```python
from build123d import *

# Parameters (mm, degrees)
BOSS_EXTRUDE1_DEPTH = 2
SKETCH3_R           = 35.7
BOSS_EXTRUDE2_DEPTH = 18.5
SKETCH5_W           = 12
SKETCH5_H           = 10
SKETCH5_R           = 1.75
BOSS_EXTRUDE3_DEPTH = 18.5
SKETCH6_R           = 36.4
BOSS_EXTRUDE5_DEPTH = 18.5
BOSS_EXTRUDE6_DEPTH = 21.5
SKETCH8_W           = 12.454054054
SKETCH8_H           = 5
CUT_EXTRUDE1_DEPTH  = 12
SKETCH9_W           = 10
SKETCH9_H           = 3
CUT_EXTRUDE2_DEPTH  = 21
CHAMFER1_SIZE       = 0.5
FILLET1_R           = 2
CHAMFER2_SIZE       = 2
SKETCH10_W          = 14
SKETCH10_H          = 10
CUT_EXTRUDE3_DEPTH  = 13


# Some blends are built 0.0001 mm under size
with BuildPart() as part:
    # Sketch4 → Boss-Extrude1 (new body)
    with BuildSketch(Plane(origin=(0, 0, 0), x_dir=(1, 0, 0), z_dir=(0, 1, 0))):
        with BuildLine():
            Line((37, 0), (37, -58))
            Line((37, -58), (-37, -58))
            Line((-37, -58), (-37, 0))
            ThreePointArc((-37, 0), (0, 37), (37, 0))
        make_face()
        with BuildLine():
            Line((-11.5, 6.062177826), (-24.769230769, 13.056998396))
            ThreePointArc((-24.769230769, 13.056998396), (-20.089945679, 19.503694076), (-13.784615385, 24.371794737))
            Line((-13.784615385, 24.371794737), (-6.4, 11.315476128))
            ThreePointArc((-6.4, 11.315476128), (-9.327474779, 9.055286535), (-11.5, 6.062177826))
        make_face(mode=Mode.SUBTRACT)
    extrude(amount=BOSS_EXTRUDE1_DEPTH)

    # Sketch3 → Boss-Extrude2 (add)
    with BuildSketch(Plane(origin=(0, 0, 0), x_dir=(1, 0, 0), z_dir=(0, 1, 0))):
        with BuildLine():
            Line((-37, 0), (-37, -58))
            Line((-37, -58), (-35, -58))
            Line((-35, -58), (-35, -38))
            Line((-35, -38), (35, -38))
            Line((35, -38), (35, -58))
            Line((35, -58), (37, -58))
            Line((37, -58), (37, 0))
            ThreePointArc((37, 0), (0, 37), (-37, 0))
        make_face()
        with Locations(Location((0, 0, 0), (0, 0, 270))):
            Circle(SKETCH3_R, mode=Mode.SUBTRACT)
    extrude(amount=BOSS_EXTRUDE2_DEPTH)

    # Sketch5 → Boss-Extrude3 (add)
    with BuildSketch(Plane(origin=(0, 0, 0), x_dir=(1, 0, 0), z_dir=(0, 1, 0))):
        with Locations((0, 40.7)):
            Rectangle(SKETCH5_W, SKETCH5_H)
        with Locations(Location((0, 41.35, 0), (0, 0, 270))):
            Circle(SKETCH5_R, mode=Mode.SUBTRACT)
    extrude(amount=BOSS_EXTRUDE3_DEPTH)

    # Sketch6 → Boss-Extrude5 (add)
    with BuildSketch(Plane(origin=(0, 0, 0), x_dir=(-1, 0, 0), z_dir=(0, 1, 0))):
        with BuildLine():
            Line((37.4, 0), (37.4, 58))
            Line((37.4, 58), (35, 58))
            Line((35, 58), (35, 38))
            Line((35, 38), (-35, 38))
            Line((-35, 38), (-35, 58))
            Line((-35, 58), (-37.4, 58))
            Line((-37.4, 58), (-37.4, 0))
            ThreePointArc((-37.4, 0), (-28.50952425, -24.206755814), (-6.064864865, -36.904978176))
            Line((-6.064864865, -36.904978176), (6.064864865, -36.904978176))
            ThreePointArc((6.064864865, -36.904978176), (28.50952425, -24.206755814), (37.4, 0))
        make_face()
        Circle(SKETCH6_R, mode=Mode.SUBTRACT)
    extrude(amount=BOSS_EXTRUDE5_DEPTH)

    # Sketch7 → Boss-Extrude6 (add)
    with BuildSketch(Plane(origin=(0, 0, 0), x_dir=(1, 0, 0), z_dir=(0, 1, 0))):
        with BuildLine():
            Line((37.4, 0), (37.4, -58))
            Line((37.4, -58), (38.4, -58))
            Line((38.4, -58), (38.4, 0))
            ThreePointArc((38.4, 0), (29.271810995, 24.853995274), (6.227027027, 37.891742298))
            Line((6.227027027, 37.891742298), (-6.227027027, 37.891742298))
            ThreePointArc((-6.227027027, 37.891742298), (-29.271810995, 24.853995274), (-38.4, 0))
            Line((-38.4, 0), (-38.4, -58))
            Line((-38.4, -58), (-37.4, -58))
            Line((-37.4, -58), (-37.4, 0))
            ThreePointArc((-37.4, 0), (0, 37.4), (37.4, 0))
        make_face()
    extrude(amount=BOSS_EXTRUDE6_DEPTH)

    # Sketch8 → Cut-Extrude1 (cut)
    with BuildSketch(Plane(origin=(0, 0, -45.7), x_dir=(-1, 0, 0), z_dir=(0, 0, -1))):
        with Locations((0, 21)):
            Rectangle(SKETCH8_W, SKETCH8_H)
    extrude(amount=-CUT_EXTRUDE1_DEPTH, mode=Mode.SUBTRACT)

    # Sketch9 → Cut-Extrude2 (cut)
    with BuildSketch(Plane.XY.offset(38)):
        with Locations((18.2, 18.9)):
            Rectangle(SKETCH9_W, SKETCH9_H)
    extrude(amount=-CUT_EXTRUDE2_DEPTH, mode=Mode.SUBTRACT)

    # Chamfer1
    # the kernel refuses this chamfer: 0.610095567, 0.5 mm, written as the material it takes off along each edge
    with BuildSketch(Plane(origin=(6.227027027, 23.093595243, -36.87796272), x_dir=(0, 0, -1), z_dir=(0, -1, 0))) as chamfer1_piece_1:
        with BuildLine():
            Line((CHAMFER1_SIZE, 0), (-0.10779544, 0.60779544))
            ThreePointArc((-0.10779544, 0.60779544), (-0.054392136, 0.313970558), (0, 0))
            Line((0, 0), (CHAMFER1_SIZE, 0))
        make_face()
    extrude(amount=4.593595243, mode=Mode.SUBTRACT)
    with BuildSketch(Plane(origin=(-6.227027027, 23.093595243, -36.87796272), x_dir=(-0.9846341969659582, 0, 0.17462960277456552), z_dir=(0, -1, 0))) as chamfer1_piece_2:
        with BuildLine():
            Line((0.61728045, 0), (-CHAMFER1_SIZE * 0.174629602775, CHAMFER1_SIZE * 0.984634196966))
            Line((-CHAMFER1_SIZE * 0.174629602775, CHAMFER1_SIZE * 0.984634196966), (0, 0))
            ThreePointArc((0, 0), (0.318644625, 0.001272197), (0.61728045, 0))
        make_face()
    extrude(amount=4.593595243, mode=Mode.SUBTRACT)
    # the kernel refuses this chamfer: 0.610095567, 0.5 mm, written as the material it takes off along each edge
    with BuildSketch(Plane(origin=(-37.4, 21.5, 59.285841494), x_dir=(-1, 0, 0), z_dir=(0, 0, -1)), Plane(origin=(37.4, 21.5, 0), x_dir=(1, 0, 0), z_dir=(0, 0, 1))) as chamfer1_2_piece_1:
        Polygon((CHAMFER1_SIZE, 0), (0, -CHAMFER1_SIZE), (0, 0), align=None)
    extrude(amount=59.285841494, mode=Mode.SUBTRACT)
    with BuildSketch(Plane(origin=(0, 21.5, 0), x_dir=(-1, 0, 0), z_dir=(0, 0, 1))) as chamfer1_2_piece_2:
        Polygon((37.4 + CHAMFER1_SIZE, 0), (37.4, CHAMFER1_SIZE), (37.4, 0), align=None)
    revolve(axis=Axis((0, 21.5, 0), (0, -1, 0)), revolution_arc=81.44055325, mode=Mode.SUBTRACT)
    with BuildSketch(Plane(origin=(0, 21.5, 0), x_dir=(0.14883547640098224, 0, -0.9888619726556849), z_dir=(-0.9888619726556849, 0, -0.14883547640098224))) as chamfer1_2_piece_3:
        Polygon((37.4 + CHAMFER1_SIZE, 0), (37.4, CHAMFER1_SIZE), (37.4, 0), align=None)
    revolve(axis=Axis((0, 21.5, 0), (0, -1, 0)), revolution_arc=81.44055325, mode=Mode.SUBTRACT)

    # Fillet1
    fillet1_edges = [part.edges().sort_by_distance(p)[0] for p in [
        (6, 0, -41.795871149),
        (18.2, 17.4, 38),
        (0, 2, 38),
        (-35, 2, 48),
        (35, 2, 48),
        (-35, 10.25, 38),
        (35, 10.25, 38),
        (-6, 0, -41.795871149),
        (-6, 9.25, -45.7),
        (6, 9.25, -45.7),
        (0, 0, -45.7),
    ]]
    fillet(fillet1_edges, radius=FILLET1_R)

    # Chamfer2
    chamfer2_edges = [part.edges().sort_by_distance(p)[0] for p in [
        (-20.089945679, 2, -19.503694076),
        (-9.327474779, 2, -9.055286535),
    ]]
    chamfer(chamfer2_edges, length=CHAMFER2_SIZE - 0.0001)  # a hair under: the kernel refuses the full size

    # Sketch10 → Cut-Extrude3 (cut)
    with BuildSketch(Plane(origin=(0, 0, 0), x_dir=(1, 0, 0), z_dir=(0, 1, 0))):
        with Locations((21, -48)):
            Rectangle(SKETCH10_W, SKETCH10_H)
    extrude(amount=CUT_EXTRUDE3_DEPTH, mode=Mode.SUBTRACT)


solid = part.part
```
The listing builds one solid part. Answer for the finished solid, in the listing's coordinates (mm). A direction names the side the tool comes from. Coordinates: 2 decimals unless noted, no trailing zeros. Loops run counter-clockwise (first coordinate to the right, second up) from the corner with the lowest first, then second, coordinate; pieces in that order, holes last. Notation, with made-up numbers: (8, -15) - (27, -15) arc R10 ccw to (27, 0) - close; hole circle Ø8 at (59.25, -31). An arc over 180 degrees is marked (long way). Use a Markdown table: item, result. Add a question column.
1) The part is cut by section A-A, the plane x = 0. Give the vertices of the cut face in (y, z).
2) The part is cut by section C-C, the plane z = -41.35. Give the vertices of the cut face in (x, y), and give its area (3 significant figures).
3) Find the intervals of material crossed by line 1 (X direction, y = 7.75, z = -41.35); line 2 (X direction, y = 8.75, z = 0); line 3 (Y direction, x = -7, z = 53), in increasing order.
4) The part is cut by section D-D, the plane z = 16. Give the vertices of the cut face in (x, y), and give its area (3 significant figures).
5) For faces 1 (the cylindrical face through (1.57, 10.134, -35.665)), 2 (the flat face through (-37.4, 20, 29)), 3 (the flat face through (0, 10, -45.7)), determine the directions among +Z, -Z, +X, -X, +Y, -Y from which every point of the face is accessible in a straight line to the end or side of a thin tool.
6) Given pin 1 (3 mm diameter, centred on y = 14, z = -41.5, fed in from -X); pin 2 (6 mm diameter, centred on x = 8.5, y = 17, fed in from -Z); pin 3 (10 mm diameter, centred on x = -5, z = 40.5, fed in from +Y), each flat-ended and moving along its own axis, determine where each tip first touches the part or whether it passes through.
7) The mould has two halves that part along Z. Classify faces 4 (the conical face through (-21, 1, -20)), 5 (the cylindrical face through (-29.025, 10.599, -25.141)), 6 (the cylindrical face through (34.43, 2.6, 49.13)): released by +Z, released by -Z, zero draft, split by the parting line, or undercut.
Here are the results:
| question | item | result |
|---|---|---|
| 1 | outline | (0, -43.7) arc R2 ccw to (2, -45.7) - (18.5, -45.7) - (18.5, -43.1) - (0, -43.1) - close; (0, -39.6) - (18.5, -39.6) - (18.5, -35.7) - (2, -35.7) - (2, 35.7) - (18.5, 35.7) - (18.5, 38) - (4, 38) arc R2 cw to (2, 40) - (2, 58) - (0, 58) - close |
| 2 | outline | (-6, 2) arc R2 ccw to (-4, 0) - (-1.75, 0) - (-1.75, 18.5) - (-6, 18.5) - close; (1.75, 0) - (4, 0) arc R2 ccw to (6, 2) - (6, 18.5) - (1.75, 18.5) - close |
| 2 | area | 156 mm^2 |
| 3 | line 1 | x = -6 to -1.75, 1.75 to 6 |
| 3 | line 2 | x = -38.4 to -35.7, 35.7 to 38.4 |
| 3 | line 3 | y = 0 to 2 |
| 4 | outline | (-38.4, 0) - (38.4, 0) - (38.4, 21.5) - (37.9, 21.5) - (37.4, 21) - (37.4, 18.5) - (31.91, 18.5) - (31.91, 2) - (-31.91, 2) - (-31.91, 18.5) - (-37.4, 18.5) - (-37.4, 21) - (-37.9, 21.5) - (-38.4, 21.5) - close |
| 4 | area | 373 mm^2 |
| 5 | face 1 | +Y |
| 5 | face 2 | +Z, +Y |
| 5 | face 3 | -Z, +X, -X, +Y, -Y |
| 6 | pin 1 | stops at x = -6 |
| 6 | pin 2 | stops at z = -45.02 |
| 6 | pin 3 | stops at y = 18.5 |
| 7 | face 4 | undercut |
| 7 | face 5 | released by -Z |
| 7 | face 6 | zero draft |
